For this review, take the finished solid that the model builds, in its own axes (mm). A direction names the side the tool comes from. Round coordinates to 2 decimals unless told otherwise and drop trailing zeros. Order: outer loops, then holes, each group sorted by start corner. A loop starts at its lowest first (then second) coordinate and runs counter-clockwise, first axis right, second up. Notation, with made-up numbers: M -22,84 L 33,84 A24 ccw 33,115 Z; hole C 47,75.5 d6. An arc over 180 degrees is marked long. Use a Markdown table: item, result.
from build123d import *

# Parameters (mm, degrees)
F0_W     = 647.936674
F0_H     = 424.298402
F1_DEPTH = 440
F0_W_2   = 660
F0_H_2   = 440
F2_DEPTH = 20


with BuildPart() as f1:
    # F0 (on Top) → F1 (new body)
    with BuildSketch(Plane.XY):
        Rectangle(F0_W, F0_H)
    extrude(amount=-F1_DEPTH)

    # F0 (on Top) → F2 (join)
    with BuildSketch(Plane.XY):
        Rectangle(F0_W_2, F0_H_2)
        Rectangle(F0_W, F0_H, mode=Mode.SUBTRACT)
        Rectangle(F0_W, F0_H)
    extrude(amount=-F2_DEPTH)


solid = f1.part
Q1. Add section B-B (x = 107.5). Write out the cut boundary in (y, z).
Determined:
| item | result |
|---|---|
| outline | M -220,-20 L -212.15,-20 L -212.15,-440 L 212.15,-440 L 212.15,-20 L 220,-20 L 220,0 L -220,0 Z |
Q2. Add section C-C (z = -45.5). Write out the cut boundary in (x, y).
Determined:
| item | result |
|---|---|
| outline | M -323.97,-212.15 L 323.97,-212.15 L 323.97,212.15 L -323.97,212.15 Z |
Q3. Add section A-A (y = -77.5). Write out the cut boundary in (x, z), then the cut area to 3 significant figures.
Determined:
| item | result |
|---|---|
| outline | M -330,-20 L -323.97,-20 L -323.97,-440 L 323.97,-440 L 323.97,-20 L 330,-20 L 330,0 L -330,0 Z |
| area | 285,000 mm^2 |
Q4. Machinability: for faces 1 (the flat face through (-323.968, -3, -227)), 2 (the flat face through (-5, 212.149, -227)), 3 (the flat face through (323.968, -3, -227)), which of the approach directions +Z, -Z, +X, -X, +Y, -Y give a long, thin tool a straight path to every point of the face, cutting with its end or side? Answer none if there is none.
Determined:
| item | result |
|---|---|
| face 1 | -Z, -X, +Y, -Y |
| face 2 | -Z, +X, -X, +Y |
| face 3 | -Z, +X, +Y, -Y |
Q5. Wall thickness on line 1 along Y through (x, z) = (44, -404.5); line 2 along X through (y, z) = (86.5, -276): over which ranges is each line inside the solid? List them lowest first. Write a range as [from, to].
Determined:
| item | result |
|---|---|
| line 1 | y = [-212.15, 212.15] |
| line 2 | x = [-323.97, 323.97] |
Q6. Clearance check with flat-ended pins moving along their axes: pin 1 (2 mm diameter, centred on y = -53.5, z = -342, fed in from -X); pin 2 (6 mm diameter, centred on x = -107.5, z = -280, fed in from -Y); pin 3 (1 mm diameter, centred on x = -136.5, z = -242, fed in from +Y). State where each tip first meets the part, or that it passes through.
Determined:
| item | result |
|---|---|
| pin 1 | stops at x = -323.97 |
| pin 2 | stops at y = -212.15 |
| pin 3 | stops at y = 212.15 |
